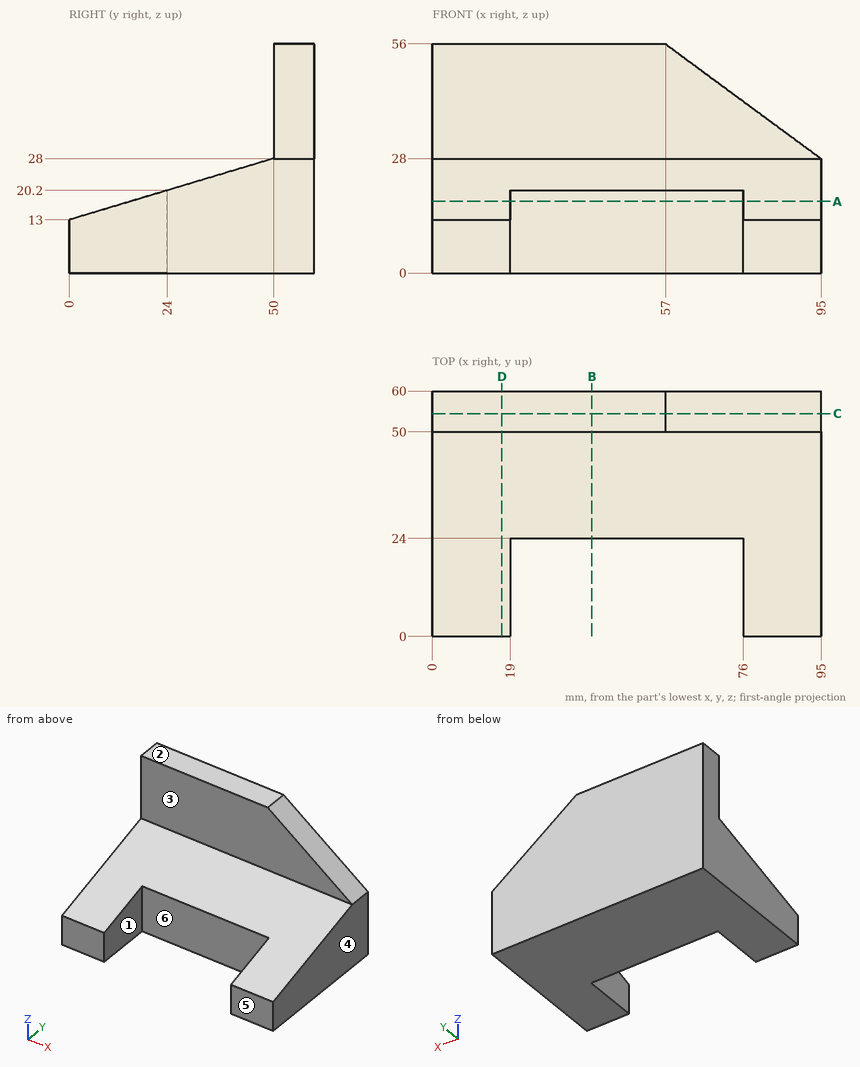
Input: dimensioned drawing with shaded views. Units: mm. Origin: part minimum x, y, z. A direction names the side the tool comes from. Coordinates: 2 decimals unless noted, no trailing zeros. Loops run counter-clockwise (first coordinate to the right, second up) from the corner with the lowest first, then second, coordinate; pieces in that order, holes last. Notation, with made-up numbers: (-26, 84) -> (30, 84) arc R17 cw to (30, 89) -> close; hole circle Ø6 at (-24.75, 61). An arc over 180 degrees is marked (long way). Use a Markdown table: item, result. Add a question column.
(1) Mould query, pull axis X, two halves, no side actions, for the marked faces 4, 5 and 6. Classes: pulls with the +X half, pulls with the -X half, needs draft (parallel to the pull), parting line crosses it, or undercut.
(2) Section query B-B, the plane x = 39. Return loops of the section in (y, z), plus the area to 3 significant figures.
(3) Line query: line 1 along Y through (x, z) = (52.5, 18); line 2 along Y through (x, z) = (51, 29.5); line 3 along Z through (x, y) = (88.5, 25.5). Output: solid intervals per line, ascending.
(4) Section query D-D, the plane x = 17. Return loops of the section in (y, z), plus the area to 4 significant figures.
(5) Pin query (flat end, axial travel): pin 1 Ø10 at (x, z) = (59.5, 5.5) entering from -Y; pin 2 Ø10 at (x, y) = (44, 23.5) entering from +Z; pin 3 Ø6 at (y, z) = (11, 12.5) entering from -X; pin 4 Ø3 at (x, y) = (46, 43) entering from +Z. Return the tip coordinate at first contact, or that it passes through.
(6) Section query A-A, the plane z = 17.5. Return loops of the section in (x, y), plus the area to 3 significant figures.
(7) Section query C-C, the plane y = 54.5. Return loops of the section in (x, z), plus the area to 3 significant figures.
(8) Access query for the marked faces 1, 2 and 3. Directions: +Z, -Z, +X, -X, +Y, -Y. A direction counts if a zero-diameter tool reaches every point of the face in a straight line with its end or side. Return the directions, or none.
Answer:
| question | item | result |
|---|---|---|
| 1 | face 4 | pulls with the +X half |
| 1 | face 5 | needs draft |
| 1 | face 6 | undercut |
| 2 | outline | (24, 0) -> (60, 0) -> (60, 56) -> (50, 56) -> (50, 28) -> (24, 20.2) -> close |
| 2 | area | 1,190 mm^2 |
| 3 | line 1 | y = 24 to 60 |
| 3 | line 2 | y = 50 to 60 |
| 3 | line 3 | z = 0 to 20.65 |
| 4 | outline | (0, 0) -> (60, 0) -> (60, 56) -> (50, 56) -> (50, 28) -> (0, 13) -> close |
| 4 | area | 1,585 mm^2 |
| 5 | pin 1 | stops at y = 24 |
| 5 | pin 2 | stops at z = 21.55 |
| 5 | pin 3 | stops at x = 0 |
| 5 | pin 4 | stops at z = 26.35 |
| 6 | outline | (0, 15) -> (19, 15) -> (19, 24) -> (76, 24) -> (76, 15) -> (95, 15) -> (95, 60) -> (0, 60) -> close |
| 6 | area | 3,760 mm^2 |
| 7 | outline | (0, 0) -> (95, 0) -> (95, 28) -> (57, 56) -> (0, 56) -> close |
| 7 | area | 4,790 mm^2 |
| 8 | face 1 | +Z, -Z, -Y |
| 8 | face 2 | +Z, +X, -X, +Y, -Y |
| 8 | face 3 | +Z, +X, -X, -Y |
